Check sheet for the modelled part. Datum: model origin and axes. Units: mm. Face numbers are marked on the shaded views. A direction names the side the tool comes from. Round coordinates to 2 decimals unless told otherwise and drop trailing zeros. Write each loop counter-clockwise with the first axis right and the second up, starting at its lowest first coordinate (ties: lowest second). Pieces come first, ordered by that corner, then holes.
Item 1: Tool access check on the marked faces 1, 2, 3 and 4. Record the directions out of +Z, -Z, +X, -X, +Y, -Y that give a thin tool (end or side, any length) a straight path to the whole face; none if there is none.
Item 2: Cross-section at C-C on y = -5. Enter the section's corners in (x, z) (3 decimals).
Item 3: Cross-section at D-D on x = -0.25. Enter the section's corners in (y, z), plus the area to 3 significant figures.
Item 4: Material ranges on line 1 (Z direction, x = 8.75, y = -5); line 2 (Z direction, x = -10.25, y = -4.75); line 3 (Z direction, x = 3, y = -3.75), recorded low to high.
Item 5: Cross-section at B-B on x = 8. Enter the section's corners in (y, z), plus the area to 3 significant figures.
Item 6: Cross-section at A-A on z = -12. Enter the section's corners in (x, y), plus the area to 3 significant figures.
Item 7: Release check for a two-part mould opening along Z. For the marked faces 5, 6 and 7 record: +Z half, -Z half, draft (parallel to the pull), parting line (faces both ways), or undercut.
Item 8: Go/stop test with flat-tipped pins: pin 1 Ø1.9 at (y, z) = (-3, -12.5) entering from -X; pin 2 Ø0.8 at (x, y) = (11.5, -4.5) entering from -Z; pin 3 Ø1.9 at (y, z) = (-3.5, 1) entering from +X. Record where each tip stops, or that it passes through.
from build123d import *

# Parameters (mm, degrees)
F0_W     = 6.35
F0_H     = 6.35
F1_DEPTH = 6.35
F2_DEPTH = 6.35


with BuildPart() as f1:
    # F0 (on Front) → F1 (new body)
    with BuildSketch(Plane.XZ):
        Polygon((-3.175, 15.345833), (-12.7, 15.345833), (-12.7, 5.820833), (-6.35, 5.820833), (-6.35, -0.529167), (-12.7, -0.529167), (-12.7, -10.054167), (-10.16, -10.054167), (-3.81, -10.054167), (3.81, -10.054167), (10.16, -10.054167), (12.7, -10.054167), (12.7, -0.529167), (6.35, -0.529167), (6.35, 5.820833), (12.7, 5.820833), (12.7, 15.345833), (3.175, 15.345833), align=None)
        with Locations((0, 18.520833)):
            Rectangle(F0_W, F0_H)
        with Locations((-9.525, 2.645833)):
            Rectangle(F0_W, F0_H)
        with Locations((9.525, 2.645833)):
            Rectangle(F0_W, F0_H)
        with Locations((-6.985, -13.229167)):
            Rectangle(F0_W, F0_H)
        with Locations((6.985, -13.229167)):
            Rectangle(F0_W, F0_H)
    extrude(amount=F1_DEPTH)

    # F0 (on Front) → F2 (cut)
    with BuildSketch(Plane.XZ):
        with Locations((-9.525, 2.645833)):
            Rectangle(F0_W, F0_H)
        with Locations((9.525, 2.645833)):
            Rectangle(F0_W, F0_H)
    extrude(amount=F2_DEPTH, mode=Mode.SUBTRACT)


solid = f1.part
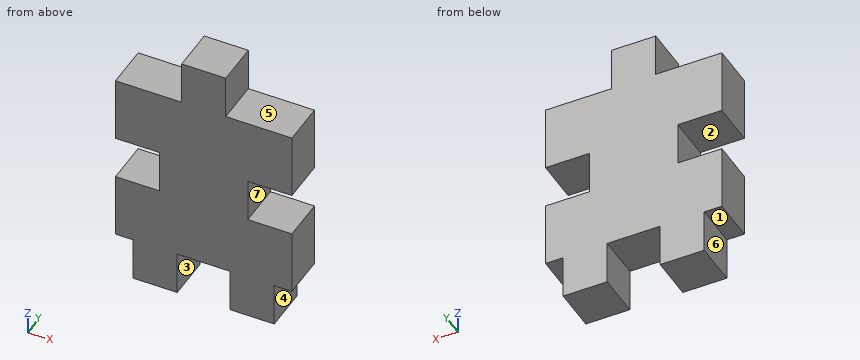
Response values:
1. face 1: -Z, -X, +Y, -Y
1. face 2: -X, +Y, -Y
1. face 3: -Z, +Y, -Y
1. face 4: -Z, +X, +Y, -Y
2. outline: (-12.7, -10.054) - (-10.16, -10.054) - (-10.16, -16.404) - (-3.81, -16.404) - (-3.81, -10.054) - (3.81, -10.054) - (3.81, -16.404) - (10.16, -16.404) - (10.16, -10.054) - (12.7, -10.054) - (12.7, -0.529) - (6.35, -0.529) - (6.35, 5.821) - (12.7, 5.821) - (12.7, 15.346) - (3.175, 15.346) - (3.175, 21.696) - (-3.175, 21.696) - (-3.175, 15.346) - (-12.7, 15.346) - (-12.7, 5.821) - (-6.35, 5.821) - (-6.35, -0.529) - (-12.7, -0.529) - close
3. outline: (-6.35, -10.05) - (0, -10.05) - (0, 21.7) - (-6.35, 21.7) - close
3. area: 202 mm2
4. line 1: z = -16.4 to -0.53, 5.82 to 15.35
4. line 2: z = -10.05 to -0.53, 5.82 to 15.35
4. line 3: z = -10.05 to 21.7
5. outline: (-6.35, -16.4) - (0, -16.4) - (0, -0.53) - (-6.35, -0.53) - close; (-6.35, 5.82) - (0, 5.82) - (0, 15.35) - (-6.35, 15.35) - close
5. area: 161 mm2
6. outline: (-10.16, -6.35) - (-3.81, -6.35) - (-3.81, 0) - (-10.16, 0) - close; (3.81, -6.35) - (10.16, -6.35) - (10.16, 0) - (3.81, 0) - close
6. area: 80.6 mm2
7. face 5: +Z half
7. face 6: draft
7. face 7: undercut
8. pin 1: stops at x = -10.16
8. pin 2: stops at z = -10.05
8. pin 3: stops at x = 6.35
